Geometry: final body of the model. Coordinates: model frame, mm. A direction names the side the tool comes from. Coordinates: 2 decimals unless noted, no trailing zeros. Loops run counter-clockwise (first coordinate to the right, second up) from the corner with the lowest first, then second, coordinate; pieces in that order, holes last. Notation, with made-up numbers: (89, -27.75) - (102, -27.75) arc R22 cw to (102, 3.25) - close; hole circle Ø7 at (84.25, 19.5). An arc over 180 degrees is marked (long way). Answer in a Markdown table with one row per item.
from build123d import *

# Parameters (mm, degrees)
ESQUISSE1_W             = 7
ESQUISSE1_H             = 7
BOSS_EXTRU_1_DEPTH      = 5.6
ESQUISSE2_W             = 4.5
ESQUISSE2_H             = 4.5
ENL_V_MAT_EXTRU_1_DEPTH = 1.6
ESQUISSE3_R             = 1.15
ENL_V_MAT_EXTRU_2_DEPTH = 11.6


with BuildPart() as part:
    # Esquisse1 → Boss.-Extru.1 (new body)
    with BuildSketch(Plane.XY):
        with Locations((3.5, 3.5)):
            Rectangle(ESQUISSE1_W, ESQUISSE1_H)
    extrude(amount=BOSS_EXTRU_1_DEPTH)

    # Esquisse2 → Enlèv. mat.-Extru.1 (cut)
    with BuildSketch(Plane.XY):
        with Locations((2.25, 2.25)):
            Rectangle(ESQUISSE2_W, ESQUISSE2_H)
    extrude(amount=ENL_V_MAT_EXTRU_1_DEPTH, mode=Mode.SUBTRACT)

    # Esquisse3 → Enlèv. mat.-Extru.2 (cut)
    with BuildSketch(Plane.XY):
        with Locations((2, 2)):
            Circle(ESQUISSE3_R)
    extrude(amount=ENL_V_MAT_EXTRU_2_DEPTH, mode=Mode.SUBTRACT)


solid = part.part
(1) Cut plane D-D on y = 0.5. Output: boundary loops of the cut face in (x, z), then the cut area to 3 significant figures.
Verdict:
| item | result |
|---|---|
| outline | (0, 1.6) - (4.5, 1.6) - (4.5, 0) - (7, 0) - (7, 5.6) - (0, 5.6) - close |
| area | 32.0 mm² |
(2) Access query for faces 4 (the face through (2, 4.5, 1)), 5 (the face through (0, 3, 3)). Directions: +Z, -Z, +X, -X, +Y, -Y. A direction counts if a zero-diameter tool reaches every point of the face in a straight line with its end or side. Return the directions, or none.
Verdict:
| item | result |
|---|---|
| face 4 | -Z, -X, -Y |
| face 5 | +Z, -Z, -X, +Y, -Y |
(3) Pull-direction query (X, two-part tool) for faces 1 (the face through (2.2, 3.3, 1.6)), 2 (the face through (7, 3, 3)), 3 (the face through (2.53, 0.98, 3.57)); classes: pulls with the +X half, pulls with the -X half, needs draft (parallel to the pull), parting line crosses it, or undercut.
Verdict:
| item | result |
|---|---|
| face 1 | needs draft |
| face 2 | pulls with the +X half |
| face 3 | undercut |
(4) Cut plane A-A on y = 2. Output: boundary loops of the cut face in (x, z), then the cut area to 3 significant figures.
Verdict:
| item | result |
|---|---|
| outline | (0, 1.6) - (0.85, 1.6) - (0.85, 5.6) - (0, 5.6) - close; (3.15, 1.6) - (4.5, 1.6) - (4.5, 0) - (7, 0) - (7, 5.6) - (3.15, 5.6) - close |
| area | 22.8 mm² |
(5) Ray query, probe 1 along X at (y, z) = (2, 3.55); probe 2 along X at (y, z) = (2, 0.5). Return the intervals inside material, ascending.
Verdict:
| item | result |
|---|---|
| probe 1 | x = 0 to 0.85, 3.15 to 7 |
| probe 2 | x = 4.5 to 7 |
(6) First-contact query: pin 1 Ø0.5 at (x, z) = (2, 1) entering from -Y; pin 2 Ø3.5 at (x, y) = (2.5, 2.5) entering from -Z; pin 3 Ø1.3 at (y, z) = (2, 0.5) entering from -X. Flat tips, straight axial feed; report the tip coordinate or a pass-through.
Verdict:
| item | result |
|---|---|
| pin 1 | stops at y = 4.5 |
| pin 2 | stops at z = 1.6 |
| pin 3 | stops at x = 4.5 |
(7) Cut plane C-C on z = 2.75. Output: boundary loops of the cut face in (x, y), then the cut area to 3 significant figures.
Verdict:
| item | result |
|---|---|
| outline | (0, 0) - (7, 0) - (7, 7) - (0, 7) - close; hole circle Ø2.3 at (2, 2) |
| area | 44.8 mm² |
